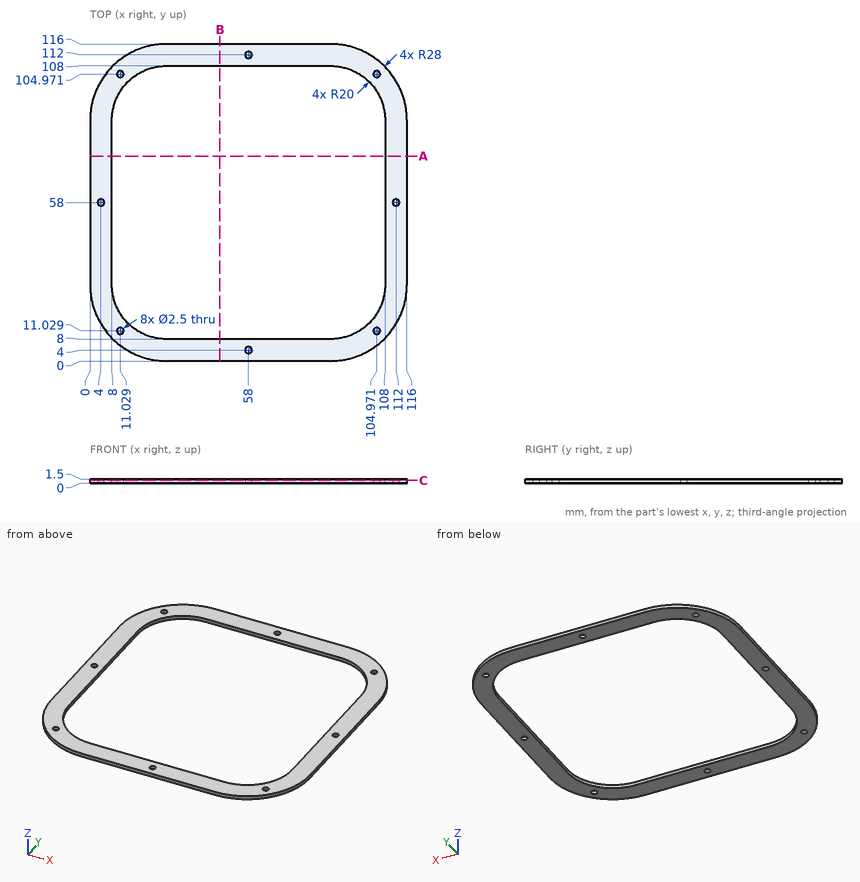
Study the drawing (mm; zero at the part's minimum x, y, z) and answer. Round coordinates to 2 decimals unless told otherwise and drop trailing zeros. Write each loop counter-clockwise with the first axis right and the second up, starting at its lowest first coordinate (ties: lowest second). Pieces come first, ordered by that corner, then holes. Notation, with made-up numbers: (70, -9) -> (112, -9) arc R28 cw to (112, 21) -> close; hole circle Ø4 at (-30, 66.5). An arc over 180 degrees is marked (long way). Use CSV: the item, a comma, the result in double quotes. Start each with the question number.
(1) Section A-A on y = 75 is taken. Give the vertices of the cut face in (x, z), then the cut area to 3 significant figures.
(2) This flat-tipped pin is pushed along its axis until it touches: pin 1 (1.5 mm diameter, centred on x = 4, y = 58, fed in from -Z). Where does it stop, or does it pass through?
(3) Section C-C on z = 1 is taken. Count the separate pieces of the cut face and the enclosed holes in it, then the cut area to 3 significant figures.
(4) Consider L1, parallel to Y at x = 34, z = 0.8; L2, parallel to Y at x = 103.5, z = 1. Determine where each line is inside the solid, lowest interval first. Write a range as from..to.
A:
1,outline,"(0, 0) -> (8, 0) -> (8, 1.5) -> (0, 1.5) -> close; (108, 0) -> (116, 0) -> (116, 1.5) -> (108, 1.5) -> close"
1,area,"24.0 mm²"
2,pin 1,"passes through"
3,separate pieces,"1"
3,enclosed holes,"9"
3,area,"3,090 mm²"
4,L1,"y = 0..8, 108..116"
4,L2,"y = 4.68..15.36, 100.64..111.32"
